Answer from the drawing. Dimensions are ordinates in mm from the lowest x, y and z of the part. A direction names the side the tool comes from. Round coordinates to 2 decimals unless told otherwise and drop trailing zeros. Order: outer loops, then holes, each group sorted by start corner. A loop starts at its lowest first (then second) coordinate and runs counter-clockwise, first axis right, second up. Notation, with made-up numbers: M 46,32 L 58,32 A25 cw 58,53 Z; hole C 48.25,88.5 d11. An arc over 180 degrees is marked long. Write item = value, one per line. Start each with the question number.
(1) Straight lines are drawn through the part: probe 1 along Y at (x, z) = (7, 4); probe 2 along Y at (x, z) = (5.5, 5.5); probe 3 along X at (y, z) = (25, 4.25). For each, find the intervals that lie inside material, in ascending order. Write a range as from..to.
(2) Which of the six approach directions +Z, -Z, +X, -X, +Y, -Y give full straight-line access (tool end or side, diameter ignored) to the marked faces 5, 6 and 7?
(3) For a pull along Y with two mould halves and no side action, classify the marked faces 1, 2, 3 and 4 as released by +Y, released by -Y, zero draft, split by the parting line, or undercut.
(4) A cutting plane is placed at C-C, the plane z = 6.75. Determine the outline of the cut face in (x, y).
(5) Each of these flat-tipped pins is pushed along its axis until it touches: pin 1 (1.4 mm diameter, centred on x = 5.5, z = 10.5, fed in from +Y); pin 2 (2 mm diameter, centred on x = 7.5, z = 10.5, fed in from -Y); pin 3 (4 mm diameter, centred on x = 7, y = 5, fed in from +Z); pin 4 (4.5 mm diameter, centred on y = 15, z = 2, fed in from +X). Where does it stop, or does it pass through?
(6) A cutting plane is placed at A-A, the plane x = 7. Determine the outline of the cut face in (y, z).
(7) A cutting plane is placed at D-D, the plane x = 4.5. Determine the outline of the cut face in (y, z), and give its area (3 significant figures).
(8) A cutting plane is placed at B-B, the plane y = 25. Determine the outline of the cut face in (x, z), and give its area (3 significant figures).
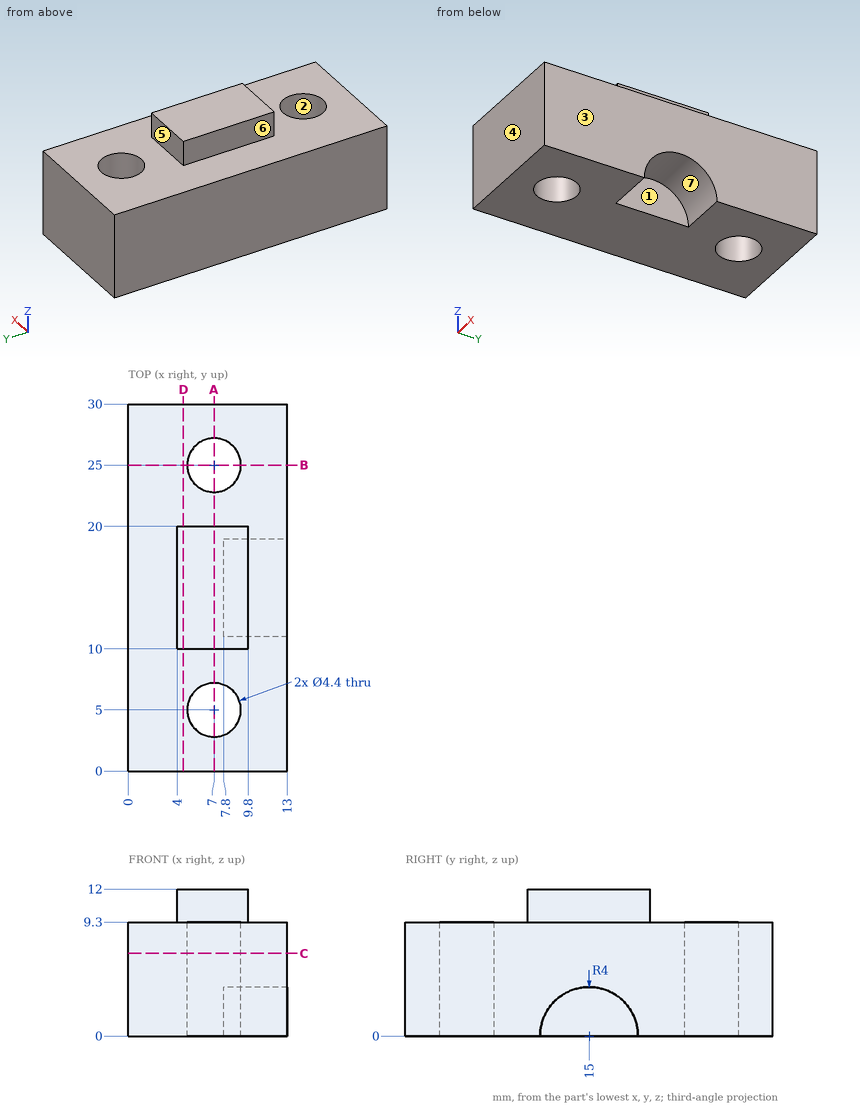
Reported:
q1.probe_1 = 0..2.8, 7.2..22.8, 27.2..30
q1.probe_2 = 0..3.39, 6.61..23.39, 26.61..30
q1.probe_3 = 0..4.8, 9.2..13
q2.face_5 = +Z, +X, -X, +Y
q2.face_6 = +Z, -X, +Y, -Y
q2.face_7 = -Z, +X
q3.face_1 = undercut
q3.face_2 = undercut
q3.face_3 = zero draft
q3.face_4 = released by -Y
q4.outline = M 0,0 L 13,0 L 13,30 L 0,30 Z; hole C 7,5 d4.4; hole C 7,25 d4.4
q5.pin_1 = 20
q5.pin_2 = 10
q5.pin_3 = through
q5.pin_4 = 13
q6.outline = M 0,0 L 2.8,0 L 2.8,9.3 L 0,9.3 Z; M 7.2,0 L 22.8,0 L 22.8,9.3 L 20,9.3 L 20,12 L 10,12 L 10,9.3 L 7.2,9.3 Z; M 27.2,0 L 30,0 L 30,9.3 L 27.2,9.3 Z
q7.outline = M 0,0 L 30,0 L 30,9.3 L 20,9.3 L 20,12 L 10,12 L 10,9.3 L 0,9.3 Z
q7.area = 306 mm²
q8.outline = M 0,0 L 4.8,0 L 4.8,9.3 L 0,9.3 Z; M 9.2,0 L 13,0 L 13,9.3 L 9.2,9.3 Z
q8.area = 80.0 mm²
